The model under review builds one solid part; all positions refer to its coordinate system, in mm. A direction names the side the tool comes from. Round coordinates to 2 decimals unless told otherwise and drop trailing zeros. Loops run counter-clockwise (first coordinate to the right, second up) from the corner with the lowest first, then second, coordinate; pieces in that order, holes last. Notation, with made-up numbers: (1.25, 36.5) -> (21.25, 36.5) arc R18 cw to (21.25, 69.5) -> close; hole circle Ø10 at (2, 41). An arc over 180 degrees is marked (long way). Return JSON: item names as keys, results as strings. Group by question number.
```python
from build123d import *

# Parameters (mm, degrees)
SKETCH1_W           = 480
SKETCH1_H           = 450
BOSS_EXTRUDE1_DEPTH = 8
SKETCH2_W           = 175
SKETCH2_H           = 100
CUT_EXTRUDE1_DEPTH  = 10
SKETCH4_R           = 3.5
BOSS_EXTRUDE3_DEPTH = 15
BOSS_EXTRUDE4_DEPTH = 90
SKETCH9_W           = 480
SKETCH9_H           = 5
BOSS_EXTRUDE6_DEPTH = 7.5
SKETCH10_W          = 480
SKETCH10_H          = 20
BOSS_EXTRUDE7_DEPTH = 2.5


with BuildPart() as part:
    # Sketch1 → Boss-Extrude1 (new body)
    with BuildSketch(Plane(origin=(0, 0, 0), x_dir=(1, 0, 0), z_dir=(0, 1, 0))):
        with Locations((240, 225)):
            Rectangle(SKETCH1_W, SKETCH1_H)
    extrude(amount=BOSS_EXTRUDE1_DEPTH)

    # Sketch2 → Cut-Extrude1 (cut)
    with BuildSketch(Plane(origin=(0, 8, 0), x_dir=(1, 0, 0), z_dir=(0, 1, 0))):
        with Locations((240, 50)):
            Rectangle(SKETCH2_W, SKETCH2_H)
    extrude(amount=-CUT_EXTRUDE1_DEPTH, mode=Mode.SUBTRACT)

    # Sketch4 → Boss-Extrude3 (add)
    with BuildSketch(Plane.XZ):
        with Locations((30, -217)):
            Circle(SKETCH4_R)
        with Locations((450, -217)):
            Circle(SKETCH4_R)
    extrude(amount=BOSS_EXTRUDE3_DEPTH)

    # Sketch5 → Boss-Extrude4 (add)
    with BuildSketch(Plane.XZ):
        Polygon((5, -445), (0, -445), (0, -450), (480, -450), (480, -445), (475, -445), align=None)
    extrude(amount=BOSS_EXTRUDE4_DEPTH)

    # Sketch9 → Boss-Extrude6 (add)
    with BuildSketch(Plane.XZ):
        with Locations((240, -370)):
            Rectangle(SKETCH9_W, SKETCH9_H)
    boss_extrude6 = extrude(amount=BOSS_EXTRUDE6_DEPTH)

    # Sketch10 → Boss-Extrude7 (add)
    with BuildSketch(Plane.XZ.offset(7.5)):
        with Locations((240, -370)):
            Rectangle(SKETCH10_W, SKETCH10_H)
    boss_extrude7 = extrude(amount=BOSS_EXTRUDE7_DEPTH)

    # Mirror9: Boss-Extrude6, Boss-Extrude7 across plane
    add(boss_extrude6.mirror(Plane.XY.offset(-315)))
    add(boss_extrude7.mirror(Plane.XY.offset(-315)))


solid = part.part
```
1. We need section B-B, the plane z = -417.5. Write out the cut boundary in (x, y).
2. We need section C-C, the plane y = -59. Write out the cut boundary in (x, z), then the cut area to 3 significant figures.
3. For P1, Ø4, axis at x = 144.5, y = -75, coming from the +Z side; P2, Ø22, axis at x = 286.5, z = -255.5, coming from the -Y side; P3, Ø9, axis at x = 281, y = 3.5, coming from the +Z side, all flat-tipped, find the tip position at first contact; note any pin that passes through.
4. Tool access review of faces 1 (the face through (480, 3, -224)), 2 (the face through (243, -44, -445)): name each direction out of +Z, -Z, +X, -X, +Y, -Y from which nothing blocks a thin tool from reaching the whole face with its end or side.
5. We need section A-A, the plane x = 348.5. Write out the cut boundary in (y, z), then the cut area to 4 significant figures.
6. Wall thickness on line 1 (Z direction, x = 83, y = -7); line 2 (Y direction, x = 443, z = -365); line 3 (Z direction, x = 295.5, y = -43): over which ranges is each line inside the solid? List them lowest first.
Check sheet entries:
{
 "1": {"outline": "(0, 0) -> (480, 0) -> (480, 8) -> (0, 8) -> close"},
 "2": {"outline": "(0, -450) -> (480, -450) -> (480, -445) -> (0, -445) -> close", "area": "2,400 mm²"},
 "3": {"P1": "stops at z = -445", "P2": "stops at y = -10", "P3": "stops at z = -100"},
 "4": {"face 1": "+Z, -Z, +X, +Y, -Y", "face 2": "+X, -X, -Y"},
 "5": {"outline": "(-90, -450) -> (8, -450) -> (8, 0) -> (0, 0) -> (0, -257.5) -> (-7.5, -257.5) -> (-7.5, -250) -> (-10, -250) -> (-10, -270) -> (-7.5, -270) -> (-7.5, -262.5) -> (0, -262.5) -> (0, -367.5) -> (-7.5, -367.5) -> (-7.5, -360) -> (-10, -360) -> (-10, -380) -> (-7.5, -380) -> (-7.5, -372.5) -> (0, -372.5) -> (0, -445) -> (-90, -445) -> close", "area": "4,225 mm²"},
 "6": {"line 1": "z = -450 to -445, -372.5 to -367.5, -262.5 to -257.5", "line 2": "y = -10 to -7.5, 0 to 8", "line 3": "z = -450 to -445"}
}
